Input: part model. Units: mm. Frame: model coordinates. A direction names the side the tool comes from. Coordinates: 2 decimals unless noted, no trailing zeros. Write each loop counter-clockwise with the first axis right and the second up, starting at its lowest first coordinate (ties: lowest second). Pieces come first, ordered by that corner, then holes. Notation, with made-up numbers: M 16,27.25 L 28,27.25 A24 ccw 28,53.25 Z; hole C 58,88 d6. An arc over 180 degrees is marked long. Answer as a JSON object with one key per item and string values. Group by question number.
from build123d import *

# Parameters (mm, degrees)
BOSS_EXTRUDE1_DEPTH     = 3
BOSS_EXTRUDE2_DEPTH     = 3
CUT_EXTRUDE1_DEPTH      = 164.987660837
CUT_EXTRUDE1_DEPTH_BACK = 164.987660837
SKETCH9_R               = 4


with BuildPart() as part:
    # Sketch7 → Boss-Extrude1 (new body)
    with BuildSketch(Plane.XY):
        Polygon((-78.549032868, 130.117059275), (38.237763696, 13.33026271), (38.237763696, -7.882940725), (17.02456026, -7.882940725), (-99.762236304, 108.903855839), (-99.762236304, 130.117059275), align=None)
    extrude(amount=BOSS_EXTRUDE1_DEPTH)

    # Sketch8 → Boss-Extrude2 (add)
    with BuildSketch(Plane.XY):
        Polygon((-78.549032868, -7.882940725), (38.237763696, 108.903855839), (38.237763696, 130.117059275), (17.02456026, 130.117059275), (-99.762236304, 13.33026271), (-99.762236304, -7.882940725), align=None)
    extrude(amount=BOSS_EXTRUDE2_DEPTH)

    # Sketch9 → Cut-Extrude1 (cut, two sides: drawn at the far end of the back side and taken through both)
    with BuildSketch(Plane.XY.offset(3).offset(-CUT_EXTRUDE1_DEPTH_BACK)):
        with Locations((-30.762236304, 61.117059275)):
            Circle(SKETCH9_R)
    extrude(amount=CUT_EXTRUDE1_DEPTH + CUT_EXTRUDE1_DEPTH_BACK, mode=Mode.SUBTRACT)


solid = part.part
Q1. Line query: line 1 (Y direction, x = 5.5, z = 2.35); line 2 (X direction, y = 59, z = 1.75); line 3 (Y direction, x = -84, z = 1.45). Output: solid intervals per line, ascending. Write a range as from..to.
Q2. Section B-B, the plane y = 1.5. Return the cut outline in (x, z).
Q3. Section A-A, the plane z = 0.8. Return the cut outline in (x, y), and give its area (3 significant figures).
Q4. Pin query (flat end, axial travel): pin 1 Ø5 at (x, y) = (19.5, 84) entering from +Z; pin 2 Ø1 at (y, z) = (55.5, 2) entering from +X. Return the tip coordinate at first contact, or that it passes through.
Q5. Draft query along X for faces 6 (the flat face through (28, -7.883, 1)), 7 (the flat face through (14.01, 84.676, 1.479)), 8 (the flat face through (-6.534, 15.676, 1.479)). Return one class per face: released by +X, released by -X, zero draft, split by the parting line, or undercut.
Q6. Access query for faces 1 (the flat face through (-54.99, 15.676, 1.479)), 2 (the flat face through (-75.53, 37.56, 1.48)), 3 (the flat face through (28, 130.117, 1)), 4 (the flat face through (-54.99, 106.56, 1.48)), 5 (the flat face through (14.01, 37.56, 1.48)). Directions: +Z, -Z, +X, -X, +Y, -Y. A direction counts if a zero-diameter tool reaches every point of the face in a straight line with its end or side. Return the directions, or none.
Q7. Section C-C, the plane x = -74. Return the cut outline in (y, z).
Q8. Section D-D, the plane y = 50.5. Return the cut outline in (x, z).
Filled in:
{
 "1": {"line 1": "3.64..46.07, 76.17..118.59", "line 2": "-54.09..-34.16, -27.37..-7.43", "line 3": "-7.88..29.09, 93.14..130.12"},
 "2": {"outline": "M -99.76,0 L -69.17,0 L -69.17,3 L -99.76,3 Z; M 7.64,0 L 38.24,0 L 38.24,3 L 7.64,3 Z"},
 "3": {"outline": "M -99.76,-7.88 L -78.55,-7.88 L -30.76,39.9 L 17.02,-7.88 L 38.24,-7.88 L 38.24,13.33 L -9.55,61.12 L 38.24,108.9 L 38.24,130.12 L 17.02,130.12 L -30.76,82.33 L -78.55,130.12 L -99.76,130.12 L -99.76,108.9 L -51.98,61.12 L -99.76,13.33 Z; hole C -30.76,61.12 d8", "area": "9,860 mm^2"},
 "4": {"pin 1": "through", "pin 2": "x = -3.43"},
 "5": {"face 6": "zero draft", "face 7": "released by +X", "face 8": "undercut"},
 "6": {"face 1": "+Z, -Z, -Y", "face 2": "+Z, -Z, -X", "face 3": "+Z, -Z, +X, -X, +Y", "face 4": "+Z, -Z, +Y", "face 5": "+Z, -Z, +X"},
 "7": {"outline": "M -3.33,0 L 39.09,0 L 39.09,3 L -3.33,3 Z; M 83.14,0 L 125.57,0 L 125.57,3 L 83.14,3 Z"},
 "8": {"outline": "M -62.59,0 L 1.07,0 L 1.07,3 L -62.59,3 Z"}
}
